```python
from build123d import *

# Parameters (mm, degrees)
SKETCH1_W           = 150
SKETCH1_H           = 200
BOSS_EXTRUDE1_DEPTH = 5
CUT_EXTRUDE1_REACH  = 7
SKETCH2_R           = 10.25
SKETCH2_R_2         = 2.65
SKETCH3_R           = 1.5
SKETCH3_R_2         = 6.5
SKETCH3_R_3         = 2.75
SKETCH3_W           = 71
SKETCH3_H           = 25
SKETCH3_W_2         = 45
SKETCH3_H_2         = 5
SKETCH3_W_3         = 13
SKETCH3_H_3         = 19
CUT_EXTRUDE2_DEPTH  = 10
SKETCH4_W           = 77.871217223
SKETCH4_H           = 8.196970234
BOSS_EXTRUDE2_DEPTH = 15
SKETCH5_W           = 62.74414778
SKETCH5_H           = 8.82586267
CUT_EXTRUDE3_DEPTH  = 15


with BuildPart() as part:
    # Sketch1 → Boss-Extrude1 (new body)
    with BuildSketch(Plane(origin=(0, 0, 0), x_dir=(1, 0, 0), z_dir=(0, 1, 0))):
        Rectangle(SKETCH1_W, SKETCH1_H)
    extrude(amount=BOSS_EXTRUDE1_DEPTH)

    # Sketch2 → Cut-Extrude1 (cut, up to next)
    with BuildSketch(Plane(origin=(0, 5, 0), x_dir=(1, 0, 0), z_dir=(0, 1, 0)), mode=Mode.PRIVATE) as cut_extrude1_sk1:
        with Locations((-50, 0)):
            Circle(SKETCH2_R)
    cut_extrude1_tool1 = extrude(cut_extrude1_sk1.sketch, amount=-CUT_EXTRUDE1_REACH, mode=Mode.PRIVATE) & part.part
    add(cut_extrude1_tool1.solids().sort_by_distance((-50, 5, 0))[0], mode=Mode.SUBTRACT)
    # Sketch2 → Cut-Extrude1 (cut, up to next)
    with BuildSketch(Plane(origin=(0, 5, 0), x_dir=(1, 0, 0), z_dir=(0, 1, 0)), mode=Mode.PRIVATE) as cut_extrude1_sk2:
        with Locations((56.7, 82.4)):
            Circle(SKETCH2_R_2)
    cut_extrude1_tool2 = extrude(cut_extrude1_sk2.sketch, amount=-CUT_EXTRUDE1_REACH, mode=Mode.PRIVATE) & part.part
    add(cut_extrude1_tool2.solids().sort_by_distance((56.7, 5, -82.4))[0], mode=Mode.SUBTRACT)
    # Sketch2 → Cut-Extrude1 (cut, up to next)
    with BuildSketch(Plane(origin=(0, 5, 0), x_dir=(1, 0, 0), z_dir=(0, 1, 0)), mode=Mode.PRIVATE) as cut_extrude1_sk3:
        with Locations((56.7, 57.4)):
            Circle(SKETCH2_R_2)
    cut_extrude1_tool3 = extrude(cut_extrude1_sk3.sketch, amount=-CUT_EXTRUDE1_REACH, mode=Mode.PRIVATE) & part.part
    add(cut_extrude1_tool3.solids().sort_by_distance((56.7, 5, -57.4))[0], mode=Mode.SUBTRACT)
    # Sketch2 → Cut-Extrude1 (cut, up to next)
    with BuildSketch(Plane(origin=(0, 5, 0), x_dir=(1, 0, 0), z_dir=(0, 1, 0)), mode=Mode.PRIVATE) as cut_extrude1_sk4:
        with Locations((56.7, -57.4)):
            Circle(SKETCH2_R_2)
    cut_extrude1_tool4 = extrude(cut_extrude1_sk4.sketch, amount=-CUT_EXTRUDE1_REACH, mode=Mode.PRIVATE) & part.part
    add(cut_extrude1_tool4.solids().sort_by_distance((56.7, 5, 57.4))[0], mode=Mode.SUBTRACT)
    # Sketch2 → Cut-Extrude1 (cut, up to next)
    with BuildSketch(Plane(origin=(0, 5, 0), x_dir=(1, 0, 0), z_dir=(0, 1, 0)), mode=Mode.PRIVATE) as cut_extrude1_sk5:
        with Locations((56.7, -82.4)):
            Circle(SKETCH2_R_2)
    cut_extrude1_tool5 = extrude(cut_extrude1_sk5.sketch, amount=-CUT_EXTRUDE1_REACH, mode=Mode.PRIVATE) & part.part
    add(cut_extrude1_tool5.solids().sort_by_distance((56.7, 5, 82.4))[0], mode=Mode.SUBTRACT)

    # Sketch3 → Cut-Extrude2 (cut)
    with BuildSketch(Plane(origin=(0, 5, 0), x_dir=(1, 0, 0), z_dir=(0, 1, 0))):
        with Locations((-44.086851081, 72.644212882)):
            Circle(SKETCH3_R)
        with Locations((-44.086851081, 41.644212882)):
            Circle(SKETCH3_R)
        with Locations((30.913148919, 72.644212882)):
            Circle(SKETCH3_R)
        with Locations((30.913148919, 41.644212882)):
            Circle(SKETCH3_R)
        with Locations((42.666816073, 19.175055369)):
            Circle(SKETCH3_R_2)
        with Locations((59.428143187, 0)):
            Circle(SKETCH3_R_3)
        with Locations((59.428143187, -14.52369357)):
            Circle(SKETCH3_R_3)
        with Locations((59.428143187, -35.082227639)):
            Circle(SKETCH3_R_3)
        with Locations((-6.586851081, 57.144212882)):
            Rectangle(SKETCH3_W, SKETCH3_H)
        with Locations((-2.709269151, -67.613370395)):
            Rectangle(SKETCH3_W_2, SKETCH3_H_2)
        with Locations((-59.961970151, 57.054006432)):
            Rectangle(SKETCH3_W_3, SKETCH3_H_3)
    extrude(amount=-CUT_EXTRUDE2_DEPTH, mode=Mode.SUBTRACT)

    # Sketch4 → Boss-Extrude2 (add)
    with BuildSketch(Plane(origin=(0, 5, 0), x_dir=(1, 0, 0), z_dir=(0, 1, 0))):
        with Locations((-0.074528718, -87.092808737)):
            Rectangle(SKETCH4_W, SKETCH4_H)
    extrude(amount=BOSS_EXTRUDE2_DEPTH)

    # Sketch5 → Cut-Extrude3 (cut)
    with BuildSketch(Plane.XY.offset(91.191293854)):
        with Locations((0.850191704, 9.412931335)):
            Rectangle(SKETCH5_W, SKETCH5_H)
    extrude(amount=-CUT_EXTRUDE3_DEPTH, mode=Mode.SUBTRACT)


solid = part.part
```
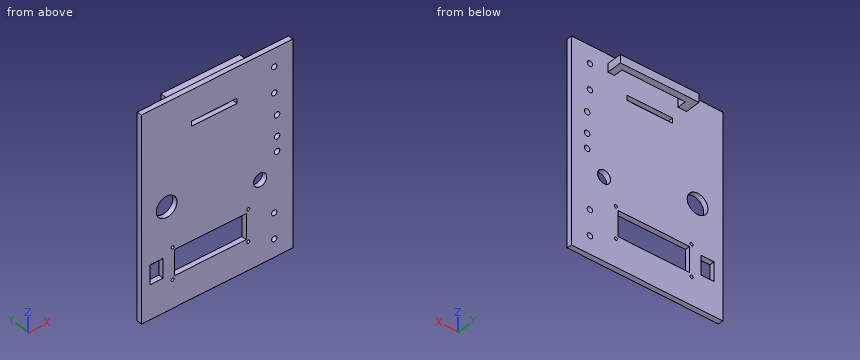
CAD build for the part. Positions are in the model's coordinates, mm. Round coordinates to 2 decimals unless told otherwise and drop trailing zeros. Write each loop counter-clockwise with the first axis right and the second up, starting at its lowest first coordinate (ties: lowest second). Pieces come first, ordered by that corner, then holes.
Item 1: Band-saw the part on C-C on x = -13.5. Write the cut outline in (y, z), then the cut area to 3 significant figures.
Filled in:
outline: (0, -100) - (5, -100) - (5, -69.64) - (0, -69.64) - close; (0, -44.64) - (5, -44.64) - (5, 65.11) - (0, 65.11) - close; (0, 70.11) - (5, 70.11) - (5, 100) - (0, 100) - close; (13.83, 82.99) - (20, 82.99) - (20, 91.19) - (13.83, 91.19) - close
area: 901 mm2
Item 2: Band-saw the part on D-D on z = 0. Write the cut outline in (x, y).
Filled in:
outline: (-75, 0) - (-60.25, 0) - (-60.25, 5) - (-75, 5) - close; (-39.75, 0) - (56.68, 0) - (56.68, 5) - (-39.75, 5) - close; (62.18, 0) - (75, 0) - (75, 5) - (62.18, 5) - close
Item 3: Band-saw the part on A-A on y = 8. Write the cut outline in (x, z).
Filled in:
outline: (-39.01, 82.99) - (-30.52, 82.99) - (-30.52, 91.19) - (-39.01, 91.19) - close; (32.22, 82.99) - (38.86, 82.99) - (38.86, 91.19) - (32.22, 91.19) - close
Item 4: Drop flat-ended pins along their axis: pin 1 Ø5 at (x, z) = (56.7, 82.4) entering from +Y; pin 2 Ø8 at (x, y) = (34.5, 13.5) entering from -Z; pin 3 Ø5 at (x, z) = (46.5, -74.5) entering from +Y. Give the stop position or say it passes through.
Filled in:
pin 1: passes through
pin 2: stops at z = 82.99
pin 3: stops at y = 5
Item 5: Band-saw the part on B-B on z = -82.4. Write the cut outline in (x, y).
Filled in:
outline: (-75, 0) - (54.05, 0) - (54.05, 5) - (-75, 5) - close; (59.35, 0) - (75, 0) - (75, 5) - (59.35, 5) - close
Item 6: Drill centre lines: L1, parallel to X at y = 2.1, z = 0; L2, parallel to Y at x = 26, z = 23; L3, parallel to X at y = 2, z = -22.5. Where is each one in solid material? Low to high.
Filled in:
L1: x = -75 to -60.25, -39.75 to 56.68, 62.18 to 75
L2: y = 0 to 5
L3: x = -75 to 37.08, 48.25 to 75
